```python
from build123d import *

# Parameters (mm, degrees)
SKETCH1_W           = 51
SKETCH1_H           = 43
SKETCH1_R           = 4.5
SKETCH1_R_2         = 1
SKETCH1_R_3         = 2
SKETCH1_R_4         = 0.5
BOSS_EXTRUDE1_DEPTH = 2.5
FILLET1_R           = 1


with BuildPart() as part:
    # Sketch1 → Boss-Extrude1 (new body)
    with BuildSketch(Plane(origin=(0, 0, 0), x_dir=(1, 0, 0), z_dir=(0, 1, 0))):
        Rectangle(SKETCH1_W, SKETCH1_H)
        with Locations(Location((0, 0, 0), (0, 0, 270))):
            Circle(SKETCH1_R, mode=Mode.SUBTRACT)
        with Locations(Location((9.7, 0, 0), (0, 0, 270))):
            Circle(SKETCH1_R_2, mode=Mode.SUBTRACT)
        with Locations(Location((-9.7, 0, 0), (0, 0, 270))):
            Circle(SKETCH1_R_2, mode=Mode.SUBTRACT)
        with Locations(Location((0, 8, 0), (0, 0, 270))):
            Circle(SKETCH1_R_2, mode=Mode.SUBTRACT)
        with Locations(Location((0, -8, 0), (0, 0, 270))):
            Circle(SKETCH1_R_2, mode=Mode.SUBTRACT)
        with Locations(Location((-10, 17.5, 0), (0, 0, 270))):
            Circle(SKETCH1_R_3, mode=Mode.SUBTRACT)
        with Locations(Location((10, 17.5, 0), (0, 0, 270))):
            Circle(SKETCH1_R_3, mode=Mode.SUBTRACT)
        with Locations(Location((-15, 0, 0), (0, 0, 270))):
            Circle(SKETCH1_R_4, mode=Mode.SUBTRACT)
        with Locations(Location((15, 0, 0), (0, 0, 270))):
            Circle(SKETCH1_R_4, mode=Mode.SUBTRACT)
        with Locations(Location((0, -17.375333522, 0), (0, 0, 270))):
            Circle(SKETCH1_R_4, mode=Mode.SUBTRACT)
        with Locations(Location((0, 15.103719109, 0), (0, 0, 270))):
            Circle(SKETCH1_R_4, mode=Mode.SUBTRACT)
        with Locations(Location((6.5, 8, 0), (0, 0, 270))):
            Circle(SKETCH1_R_4, mode=Mode.SUBTRACT)
        with Locations(Location((-6.5, 8, 0), (0, 0, 270))):
            Circle(SKETCH1_R_4, mode=Mode.SUBTRACT)
        with Locations(Location((-6.5, -8, 0), (0, 0, 270))):
            Circle(SKETCH1_R_4, mode=Mode.SUBTRACT)
        with Locations(Location((6.5, -8, 0), (0, 0, 270))):
            Circle(SKETCH1_R_4, mode=Mode.SUBTRACT)
        with BuildLine():
            Line((-20.5, -18.5), (-14.5, -18.5))
            ThreePointArc((-14.5, -18.5), (-13.085786438, -17.914213562), (-12.5, -16.5))
            Line((-12.5, -16.5), (-12.5, -10.5))
            ThreePointArc((-12.5, -10.5), (-13.085786438, -9.085786438), (-14.5, -8.5))
            Line((-14.5, -8.5), (-20.5, -8.5))
            ThreePointArc((-20.5, -8.5), (-21.914213562, -9.085786438), (-22.5, -10.5))
            Line((-22.5, -10.5), (-22.5, -16.5))
            ThreePointArc((-22.5, -16.5), (-21.914213562, -17.914213562), (-20.5, -18.5))
        make_face(mode=Mode.SUBTRACT)
    extrude(amount=BOSS_EXTRUDE1_DEPTH)

    # Fillet1
    fillet1_edges = [part.edges().sort_by_distance(p)[0] for p in [
        (25.5, 1.25, -21.5),
        (25.5, 1.25, 21.5),
        (-25.5, 1.25, 21.5),
        (-25.5, 1.25, -21.5),
    ]]
    fillet(fillet1_edges, radius=FILLET1_R)


solid = part.part
```
Geometry: final body of the model. Coordinates: model frame, mm. A direction names the side the tool comes from. Coordinates: 2 decimals unless noted, no trailing zeros. Order: outer loops, then holes, each group sorted by start corner. A loop starts at its lowest first (then second) coordinate and runs counter-clockwise, first axis right, second up. Notation, with made-up numbers: M 81.25,-15.75 L 95.25,-15.75 A27 cw 95.25,7.25 Z; hole C 1,5 d11. An arc over 180 degrees is marked long. Answer in a Markdown table with one row per item. Add a question column.
Q1. Mould query, pull axis Z, two halves, no side actions, for faces 3 (the flat face through (0, 1, 21.5)), 4 (the flat face through (-17, 1, 8.5)), 5 (the flat face through (-22.5, 1, 13)), 6 (the flat face through (-25.5, 1, 0)). Classes: released by +Z, released by -Z, zero draft, split by the parting line, or undercut.
Q2. Line query: L1, parallel to X at y = 1.3, z = 0; L2, parallel to X at y = 1.1, z = -8; L3, parallel to Z at x = -17, y = 0.9. Output: solid intervals per line, ascending.
Q3. Section query B-B on z = -17.5. Return the cut outline in (x, y), and give its area (4 significant figures).
Q4. Section query A-A on x = -18.5. Return the cut outline in (y, z), and give its area (3 significant figures).
Q5. Section query C-C on y = 1.4. Count the separate pieces of the cut face and the enclosed holes in it, and give its area (3 significant figures).
Q6. Reachability of faces 1 (the flat face through (-12.5, 1, 14)), 2 (the flat face through (25.5, 1, 0)) from +Z, -Z, +X, -X, +Y, -Y: full face, straight path, thin tool, end or side. Return the list, or none.
Q7. Contact query for a flat-ended pin moving along its axis: P1, Ø1.8, axis at x = 0, z = 8, coming from the -Y side. Output: stop coordinate, or through.
Q8. Section query D-D on x = 2.5. Return the cut outline in (y, z), and give its area (3 significant figures).
Completed:
| question | item | result |
|---|---|---|
| 1 | face 3 | released by +Z |
| 1 | face 4 | undercut |
| 1 | face 5 | undercut |
| 1 | face 6 | zero draft |
| 2 | L1 | x = -25.5 to -15.5, -14.5 to -10.7, -8.7 to -4.5, 4.5 to 8.7, 10.7 to 14.5, 15.5 to 25.5 |
| 2 | L2 | x = -25.5 to -7, -6 to -1, 1 to 6, 7 to 25.5 |
| 2 | L3 | z = -21.5 to 8.5, 18.5 to 21.5 |
| 3 | outline | M -25.5,0 L -12,0 L -12,2.5 L -25.5,2.5 Z; M -8,0 L 8,0 L 8,2.5 L -8,2.5 Z; M 12,0 L 25.5,0 L 25.5,2.5 L 12,2.5 Z |
| 3 | area | 107.5 mm2 |
| 4 | outline | M 0,-21.5 L 2.5,-21.5 L 2.5,8.5 L 0,8.5 Z; M 0,18.5 L 2.5,18.5 L 2.5,21.5 L 0,21.5 Z |
| 4 | area | 82.5 mm2 |
| 5 | separate pieces | 1 |
| 5 | enclosed holes | 16 |
| 5 | area | 1,990 mm2 |
| 6 | face 1 | +Y, -Y |
| 6 | face 2 | +Z, -Z, +X, +Y, -Y |
| 7 | P1 | passes through |
| 8 | outline | M 0,-21.5 L 2.5,-21.5 L 2.5,-3.74 L 0,-3.74 Z; M 0,3.74 L 2.5,3.74 L 2.5,21.5 L 0,21.5 Z |
| 8 | area | 88.8 mm2 |
